from build123d import *

# Parameters (mm, degrees)
F3_DEPTH = 75
F4_W     = 30
F4_H     = 42
F5_DEPTH = 25
F6_D     = 4.5
F7_R     = 10


with BuildPart() as f3:
    # F2 (on Top) → F3 (new body)
    with BuildSketch(Plane.XY):
        Polygon((0, 0), (2, 0), (2, 10), (9, 10), (9, -65), (11, -65), (11, 12), (0, 12), align=None)
    extrude(amount=F3_DEPTH)

    # F4 (on face) → F5 (cut)
    with BuildSketch(Plane.YZ.offset(11)):
        with Locations((-3, 37.5)):
            Rectangle(F4_W, F4_H)
    extrude(amount=-F5_DEPTH, mode=Mode.SUBTRACT)

    # F6 (through all)
    with Locations(Plane.YZ.offset(11)):
        with Locations((-38, 65), (-38, 10)):
            Hole(F6_D / 2)

    # F7
    f7_edges = [f3.edges().sort_by_distance(p)[0] for p in [
        (10, -65, 0),
        (10, -65, 75),
    ]]
    fillet(f7_edges, radius=F7_R)


solid = f3.part
CAD build for the part. Positions are in the model's coordinates, mm. A direction names the side the tool comes from. Round coordinates to 2 decimals unless told otherwise and drop trailing zeros. Write each loop counter-clockwise with the first axis right and the second up, starting at its lowest first coordinate (ties: lowest second). Pieces come first, ordered by that corner, then holes.
(1) Probe line 1 along Z through (x, y) = (10.55, -38); line 2 along X through (y, z) = (4.5, 71.5); line 3 along Y through (x, z) = (9.5, 40.5). List the from-to ranges inside material, lowest first.
(2) Slice it at C-C, the plane z = 14. Write the cut outline in (x, y), and give its area (3 significant figures).
(3) Drop flat-ended pins along their axis: P1, Ø1, axis at x = 1, z = 66.5, coming from the -Y side; P2, Ø1, axis at y = -11, z = 66.5, coming from the -X side; P3, Ø1.6, axis at x = 10, z = 30, coming from the +Y side; P4, Ø4, axis at x = 8, y = -32.5, coming from the -Z side. Give the stop position or say it passes through.
(4) Slice it at B-B, the plane y = 7. Write the cut outline in (x, z).
(5) Mould opens along X. For faces 4 (the face through (5, 10, 67)), 5 (the face through (0, 6, 8)), 6 (the face through (10, -65, 37)) say: pulls with the +X half, pulls with the -X half, needs draft (parallel to the pull), parting line crosses it, or undercut.
(6) 3-axis set-ups, long thin cutter, end or side, ignore diameter. For faces 1 (the face through (1, 0, 8)), 2 (the face through (2, 5, 67)), 3 (the face through (9.2, 0.1, 58.5)): which of +Z, -Z, +X, -X, +Y, -Y reach the whole face in a straight line?
(7) Slice it at A-A, the plane x = 7. Write the cut outline in (y, z), and give its area (3 significant figures).
(8) Slice it at D-D, the plane y = -1. Write the cut outline in (x, z), and give its area (3 significant figures).
From the geometry:
1. line 1: z = 0 to 7.75, 12.25 to 62.75, 67.25 to 75
1. line 2: x = 0 to 2, 9 to 11
1. line 3: y = -65 to -18
2. outline: (0, 0) - (2, 0) - (2, 10) - (9, 10) - (9, -65) - (11, -65) - (11, 12) - (0, 12) - close
2. area: 192 mm2
3. P1: stops at y = 0
3. P2: stops at x = 9
3. P3: stops at y = -18
3. P4: stops at z = 0
4. outline: (0, 0) - (2, 0) - (2, 16.5) - (0, 16.5) - close; (0, 58.5) - (2, 58.5) - (2, 75) - (0, 75) - close; (9, 0) - (11, 0) - (11, 16.5) - (9, 16.5) - close; (9, 58.5) - (11, 58.5) - (11, 75) - (9, 75) - close
5. face 4: undercut
5. face 5: pulls with the -X half
5. face 6: needs draft
6. face 1: +Z, -Z, -X, -Y
6. face 2: +Z, -Z, -Y
6. face 3: +X, -X, +Y
7. outline: (10, 0) - (12, 0) - (12, 16.5) - (10, 16.5) - close; (10, 58.5) - (12, 58.5) - (12, 75) - (10, 75) - close
7. area: 66.0 mm2
8. outline: (9, 0) - (11, 0) - (11, 16.5) - (9, 16.5) - close; (9, 58.5) - (11, 58.5) - (11, 75) - (9, 75) - close
8. area: 66.0 mm2
